from build123d import *
from OCP.BRepFilletAPI import BRepFilletAPI_MakeChamfer

# Parameters (mm, degrees)
SKETCH1_W           = 40.132
SKETCH1_H           = 21.336
BOSS_EXTRUDE1_DEPTH = 36.195
BOSS_EXTRUDE3_DEPTH = 2.54
CHAMFER1_SIZE       = 2.54
SKETCH7_R           = 2.286
BOSS_EXTRUDE4_DEPTH = 2.54
CHAMFER2_SIZE       = 3.556
CHAMFER2_SIZE2      = 2.54
CUT_EXTRUDE11_REACH = 53.909
BOSS_EXTRUDE5_DEPTH = 1.524
SKETCH14_R          = 2.159
SKETCH14_R_2        = 1.016
BOSS_EXTRUDE6_DEPTH = 2.032
SKETCH15_R          = 3.048
SKETCH15_R_2        = 1.27
BOSS_EXTRUDE7_DEPTH = 3.556
BOSS_EXTRUDE8_DEPTH = 7.62


with BuildPart() as part:
    # Sketch1 → Boss-Extrude1 (new body)
    with BuildSketch(Plane.XY):
        with Locations((-2.744373002, 5.334902309)):
            Rectangle(SKETCH1_W, SKETCH1_H)
    extrude(amount=BOSS_EXTRUDE1_DEPTH)

    # Sketch6 → Boss-Extrude3 (add)
    with BuildSketch(Plane(origin=(0, 0, 0), x_dir=(-1, 0, 0), z_dir=(0, 0, -1))):
        with BuildLine():
            Line((7.598682871, 14.986902309), (-14.273626998, 14.986902309))
            Line((-14.273626998, 14.986902309), (-14.273626998, -4.317097691))
            Line((-14.273626998, -4.317097691), (7.598682871, -4.317097691))
            ThreePointArc((7.598682871, -4.317097691), (22.810373002, 5.334902309), (7.598682871, 14.986902309))
        make_face()
    extrude(amount=BOSS_EXTRUDE3_DEPTH)

    # Chamfer1
    chamfer1_edges = [part.edges().sort_by_distance(p)[0] for p in [
        (14.273626998, 5.334902309, -2.54),
    ]]
    chamfer(chamfer1_edges, length=CHAMFER1_SIZE - 0.0001)  # a hair under: the kernel refuses the full size

    # Sketch7 → Boss-Extrude4 (add)
    with BuildSketch(Plane(origin=(0, 0, 8.89), x_dir=(-1, 0, 0), z_dir=(0, 0, -1))):
        with BuildLine():
            Line((22.810373002, 16.002902309), (22.810373002, -5.333097691))
            Line((22.810373002, -5.333097691), (31.192373002, -5.333097691))
            ThreePointArc((31.192373002, -5.333097691), (32.090398614, -4.961123303), (32.462373002, -4.063097691))
            Line((32.462373002, -4.063097691), (32.462373002, 3.359346754))
            ThreePointArc((32.462373002, 3.359346754), (31.78454458, 5.334902309), (32.462373002, 7.310457865))
            Line((32.462373002, 7.310457865), (32.462373002, 14.732902309))
            ThreePointArc((32.462373002, 14.732902309), (32.090398614, 15.630927921), (31.192373002, 16.002902309))
            Line((31.192373002, 16.002902309), (22.810373002, 16.002902309))
        make_face()
        with Locations((27.890373002, 0.762902309)):
            Circle(SKETCH7_R, mode=Mode.SUBTRACT)
        with Locations((27.890373002, 9.906902309)):
            Circle(SKETCH7_R, mode=Mode.SUBTRACT)
    boss_extrude4 = extrude(amount=BOSS_EXTRUDE4_DEPTH)

    # Mirror1: Boss-Extrude4 across plane
    add(boss_extrude4.mirror(Plane(origin=(-2.744373002, 0, 0), x_dir=(0, 0, 1), z_dir=(1, 0, 0))))

    # Chamfer2: one chamfer whose edges measure the first distance from different faces: ONE call of the kernel's chamfer builder (chamfer() names one face for all edges)
    chamfer2_edges_1 = [part.edges().sort_by_distance(p)[0] for p in [
        (17.321626998, 5.334902309, 36.195),
    ]]
    chamfer2_side_1 = [part.faces().sort_by_distance(p)[0] for p in [
        (17.321626998, 5.334902309, 22.5425),
    ]]
    chamfer2_edges_2 = [part.edges().sort_by_distance(p)[0] for p in [
        (-2.744373002, 16.002902309, 36.195),
    ]]
    chamfer2_side_2 = [part.faces().sort_by_distance(p)[0] for p in [
        (-2.744373002, 16.002902309, 17.79911165),
    ]]
    chamfer2_edges_3 = [part.edges().sort_by_distance(p)[0] for p in [
        (-2.744373002, -5.333097691, 36.195),
    ]]
    chamfer2_side_3 = [part.faces().sort_by_distance(p)[0] for p in [
        (-2.744373002, -5.333097691, 17.79911165),
    ]]
    chamfer2_edges_4 = [part.edges().sort_by_distance(p)[0] for p in [
        (-22.810373002, 5.334902309, 36.195),
    ]]
    chamfer2_side_4 = [part.faces().sort_by_distance(p)[0] for p in [
        (-22.810373002, 5.334902309, 22.5425),
    ]]
    chamfer2 = BRepFilletAPI_MakeChamfer(part.part.solid().wrapped)
    for e in chamfer2_edges_1:
        chamfer2.Add(CHAMFER2_SIZE, CHAMFER2_SIZE2, e.wrapped, chamfer2_side_1[0].wrapped)  # the first distance lies on this face
    for e in chamfer2_edges_2:
        chamfer2.Add(CHAMFER2_SIZE, CHAMFER2_SIZE2, e.wrapped, chamfer2_side_2[0].wrapped)  # the first distance lies on this face
    for e in chamfer2_edges_3:
        chamfer2.Add(CHAMFER2_SIZE, CHAMFER2_SIZE2, e.wrapped, chamfer2_side_3[0].wrapped)  # the first distance lies on this face
    for e in chamfer2_edges_4:
        chamfer2.Add(CHAMFER2_SIZE, CHAMFER2_SIZE2, e.wrapped, chamfer2_side_4[0].wrapped)  # the first distance lies on this face
    add(Compound.cast(chamfer2.Shape()), mode=Mode.REPLACE)

    # Sketch12 → Cut-Extrude11 (cut, up to next)
    with BuildSketch(Plane.XY.offset(34.671), mode=Mode.PRIVATE) as cut_extrude11_sk1:
        with BuildLine():
            Line((-21.35894443, 14.551473738), (-21.35894443, 9.979473738))
            ThreePointArc((-21.35894443, 9.979473738), (-18.126052227, 11.318581534), (-16.78694443, 14.551473738))
            Line((-16.78694443, 14.551473738), (-21.35894443, 14.551473738))
        make_face()
    cut_extrude11_tool1 = extrude(cut_extrude11_sk1.sketch, amount=CUT_EXTRUDE11_REACH, mode=Mode.PRIVATE) & part.part
    # Sketch12 → Cut-Extrude11 (cut, up to next)
    with BuildSketch(Plane.XY.offset(34.671), mode=Mode.PRIVATE) as cut_extrude11_sk2:
        with BuildLine():
            Line((15.870198427, 14.551473738), (11.298198427, 14.551473738))
            ThreePointArc((11.298198427, 14.551473738), (12.637306223, 11.318581534), (15.870198427, 9.979473738))
            Line((15.870198427, 9.979473738), (15.870198427, 14.551473738))
        make_face()
    cut_extrude11_tool2 = extrude(cut_extrude11_sk2.sketch, amount=CUT_EXTRUDE11_REACH, mode=Mode.PRIVATE) & part.part
    # Sketch12 → Cut-Extrude11 (cut, up to next)
    with BuildSketch(Plane.XY.offset(34.671), mode=Mode.PRIVATE) as cut_extrude11_sk3:
        with BuildLine():
            Line((15.870198427, -3.88166912), (15.870198427, 0.69033088))
            ThreePointArc((15.870198427, 0.69033088), (12.637306223, -0.648776916), (11.298198427, -3.88166912))
            Line((11.298198427, -3.88166912), (15.870198427, -3.88166912))
        make_face()
    cut_extrude11_tool3 = extrude(cut_extrude11_sk3.sketch, amount=CUT_EXTRUDE11_REACH, mode=Mode.PRIVATE) & part.part
    # Sketch12 → Cut-Extrude11 (cut, up to next)
    with BuildSketch(Plane.XY.offset(34.671), mode=Mode.PRIVATE) as cut_extrude11_sk4:
        with BuildLine():
            Line((-21.35894443, -3.88166912), (-16.78694443, -3.88166912))
            ThreePointArc((-16.78694443, -3.88166912), (-18.126052227, -0.648776916), (-21.35894443, 0.69033088))
            Line((-21.35894443, 0.69033088), (-21.35894443, -3.88166912))
        make_face()
    cut_extrude11_tool4 = extrude(cut_extrude11_sk4.sketch, amount=CUT_EXTRUDE11_REACH, mode=Mode.PRIVATE) & part.part
    add(cut_extrude11_tool1.solids().sort_by_distance((-19.418527, 12.611057, 34.671))[0], mode=Mode.SUBTRACT)
    add(cut_extrude11_tool2.solids().sort_by_distance((13.929781, 12.611057, 34.671))[0], mode=Mode.SUBTRACT)
    add(cut_extrude11_tool3.solids().sort_by_distance((13.929781, -1.941252, 34.671))[0], mode=Mode.SUBTRACT)
    add(cut_extrude11_tool4.solids().sort_by_distance((-19.418527, -1.941252, 34.671))[0], mode=Mode.SUBTRACT)

    # Sketch13 → Boss-Extrude5 (add)
    with BuildSketch(Plane(origin=(0, 0, -2.54), x_dir=(-1, 0, 0), z_dir=(0, 0, -1))):
        with BuildLine():
            Line((20.651373002, 7.493902309), (18.114074518, 7.493902309))
            ThreePointArc((18.114074518, 7.493902309), (16.632501062, 9.82503037), (14.301373002, 11.306603825))
            Line((14.301373002, 11.306603825), (14.301373002, 13.843902309))
            ThreePointArc((14.301373002, 13.843902309), (12.142373002, 16.002902309), (9.983373002, 13.843902309))
            Line((9.983373002, 13.843902309), (9.983373002, 11.306603825))
            ThreePointArc((9.983373002, 11.306603825), (7.652244941, 9.82503037), (6.170671485, 7.493902309))
            Line((6.170671485, 7.493902309), (3.633373002, 7.493902309))
            ThreePointArc((3.633373002, 7.493902309), (1.474373002, 5.334902309), (3.633373002, 3.175902309))
            Line((3.633373002, 3.175902309), (6.170671485, 3.175902309))
            ThreePointArc((6.170671485, 3.175902309), (7.652244941, 0.844774249), (9.983373002, -0.636799207))
            Line((9.983373002, -0.636799207), (9.983373002, -3.174097691))
            ThreePointArc((9.983373002, -3.174097691), (12.142373002, -5.333097691), (14.301373002, -3.174097691))
            Line((14.301373002, -3.174097691), (14.301373002, -0.636799207))
            ThreePointArc((14.301373002, -0.636799207), (16.632501062, 0.844774249), (18.114074518, 3.175902309))
            Line((18.114074518, 3.175902309), (20.651373002, 3.175902309))
            ThreePointArc((20.651373002, 3.175902309), (22.810373002, 5.334902309), (20.651373002, 7.493902309))
        make_face()
    extrude(amount=BOSS_EXTRUDE5_DEPTH)

    # Sketch14 → Boss-Extrude6 (add)
    # profile 1 of 4: a face of its own
    with BuildSketch(Plane(origin=(0, 0, -4.064), x_dir=(-1, 0, 0), z_dir=(0, 0, -1))):
        with Locations((12.142373002, 13.843902309)):
            Circle(SKETCH14_R)
        with Locations((12.142373002, 13.843902309)):
            Circle(SKETCH14_R_2, mode=Mode.SUBTRACT)
    # profile 2 of 4: a face of its own
    with BuildSketch(Plane(origin=(0, 0, -4.064), x_dir=(-1, 0, 0), z_dir=(0, 0, -1))):
        with Locations((20.651373002, 5.334902309)):
            Circle(SKETCH14_R)
        with Locations((20.651373002, 5.334902309)):
            Circle(SKETCH14_R_2, mode=Mode.SUBTRACT)
    # profile 3 of 4: a face of its own
    with BuildSketch(Plane(origin=(0, 0, -4.064), x_dir=(-1, 0, 0), z_dir=(0, 0, -1))):
        with Locations((12.142373002, -3.174097691)):
            Circle(SKETCH14_R)
        with Locations((12.142373002, -3.174097691)):
            Circle(SKETCH14_R_2, mode=Mode.SUBTRACT)
    # profile 4 of 4: a face of its own
    with BuildSketch(Plane(origin=(0, 0, -4.064), x_dir=(-1, 0, 0), z_dir=(0, 0, -1))):
        with Locations(Location((3.633373002, 5.334902309, 0), (0, 0, 90))):
            Circle(SKETCH14_R)
        with Locations((3.633373002, 5.334902309)):
            Circle(SKETCH14_R_2, mode=Mode.SUBTRACT)
    extrude(amount=BOSS_EXTRUDE6_DEPTH)

    # Sketch15 → Boss-Extrude7 (add)
    with BuildSketch(Plane(origin=(0, 0, -4.064), x_dir=(-1, 0, 0), z_dir=(0, 0, -1))):
        with Locations(Location((12.142373002, 5.334902309, 0), (0, 0, 180))):
            Circle(SKETCH15_R)
        with Locations(Location((12.142373002, 5.334902309, 0), (0, 0, 180))):
            Circle(SKETCH15_R_2, mode=Mode.SUBTRACT)
    extrude(amount=BOSS_EXTRUDE7_DEPTH)

    # Sketch16 → Boss-Extrude8 (add)
    with BuildSketch(Plane.ZY.offset(22.810373002)):
        with BuildLine():
            Line((27.813, 4.616481819), (27.813, 4.529322799))
            ThreePointArc((27.813, 4.529322799), (27.559, 3.048902309), (27.305, 4.529322799))
            Line((27.305, 4.529322799), (27.305, 4.616481819))
            ThreePointArc((27.305, 4.616481819), (26.797, 5.334902309), (27.305, 6.053322799))
            Line((27.305, 6.053322799), (27.305, 6.140481819))
            ThreePointArc((27.305, 6.140481819), (27.559, 7.620902309), (27.813, 6.140481819))
            Line((27.813, 6.140481819), (27.813, 6.053322799))
            ThreePointArc((27.813, 6.053322799), (28.321, 5.334902309), (27.813, 4.616481819))
        make_face()
    extrude(amount=BOSS_EXTRUDE8_DEPTH)


solid = part.part
Input: part model. Units: mm. Frame: model coordinates. A direction names the side the tool comes from. Give positions to 0.01 mm unless a question says otherwise; leave off trailing zeros. Loops run counter-clockwise (first coordinate to the right, second up) from the corner with the lowest first, then second, coordinate; pieces in that order, holes last. Notation, with made-up numbers: (55, 51) -> (82, 51) arc R28 cw to (82, 82) -> close; hole circle Ø7 at (1.25, 51.5). An arc over 180 degrees is marked (long way). Answer as a JSON object with one key per item and string values. Group by question number.
Item 1: Cut plane A-A, the plane x = -24.5. Return the cut outline in (y, z) (3 decimals).
Item 2: Reachability of faces 1 (the cylindrical face through (-20.431, 4.343, -5.066)), 2 (the flat face through (14, -2, 34.671)), 3 (the flat face through (-13, -4, -6.096)) from +Z, -Z, +X, -X, +Y, -Y: full face, straight path, thin tool, end or side. Return the list, or none.
Item 3: Cut plane C-C, the plane z = 20. Return the cut outline in (x, y).
Item 4: Pin query (flat end, axial travel): P1, Ø6, axis at y = -1.5, z = 16.5, coming from the -X side; P2, Ø10, axis at x = 4.5, y = 12, coming from the -Z side; P3, Ø4, axis at y = 1.5, z = 31, coming from the +X side. Return the tip coordinate at first contact, or that it passes through.
Item 5: Cut plane B-B, the plane x = 21. Return the cut outline in (y, z), and give its area (3 significant figures).
Item 6: Pull-direction query (Y, two-part tool) for faces 4 (the cylindrical face through (-16.66, 9.8, -3.29)), 5 (the flat face through (-28, 5, 8.89)), 6 (the flat face through (-21, 5, -4.064)); classes: released by +Y, released by -Y, zero draft, split by the parting line, or undercut.
Item 7: Line query: probe 1 along Z at (x, y) = (18.5, -0.75); probe 2 along Z at (x, y) = (10, 0) (3 decimals); probe 3 along X at (y, z) = (3.75, 32). Output: solid intervals per line, ascending.
Checks:
{
 "1": {"outline": "(-5.333, 6.35) -> (16.003, 6.35) -> (16.003, 8.89) -> (-5.333, 8.89) -> close; (4.529, 27.305) -> (4.616, 27.305) arc R0.762 ccw to (6.053, 27.305) -> (6.14, 27.305) arc R0.762 ccw (long way) to (6.14, 27.813) -> (6.053, 27.813) arc R0.762 ccw to (4.616, 27.813) -> (4.529, 27.813) arc R0.762 ccw (long way) to start"},
 "2": {"face 1": "-Z", "face 2": "+Z, +X, -Y", "face 3": "-Z, +X, -X, -Y"},
 "3": {"outline": "(-22.81, -5.33) -> (17.32, -5.33) -> (17.32, 16) -> (-22.81, 16) -> close"},
 "4": {"P1": "stops at x = -22.81", "P2": "stops at z = -2.54", "P3": "stops at x = 17.32"},
 "5": {"outline": "(-5.33, 6.35) -> (-1.04, 6.35) -> (-1.04, 8.89) -> (-5.33, 8.89) -> close; (2.57, 6.35) -> (8.1, 6.35) -> (8.1, 8.89) -> (2.57, 8.89) -> close; (11.71, 6.35) -> (16, 6.35) -> (16, 8.89) -> (11.71, 8.89) -> close", "area": "35.8 mm²"},
 "6": {"face 4": "released by +Y", "face 5": "zero draft", "face 6": "undercut"},
 "7": {"probe 1": "z = 6.35 to 8.89", "probe 2": "z = -2.54 to 36.195", "probe 3": "x = -22.81 to 17.32"}
}
